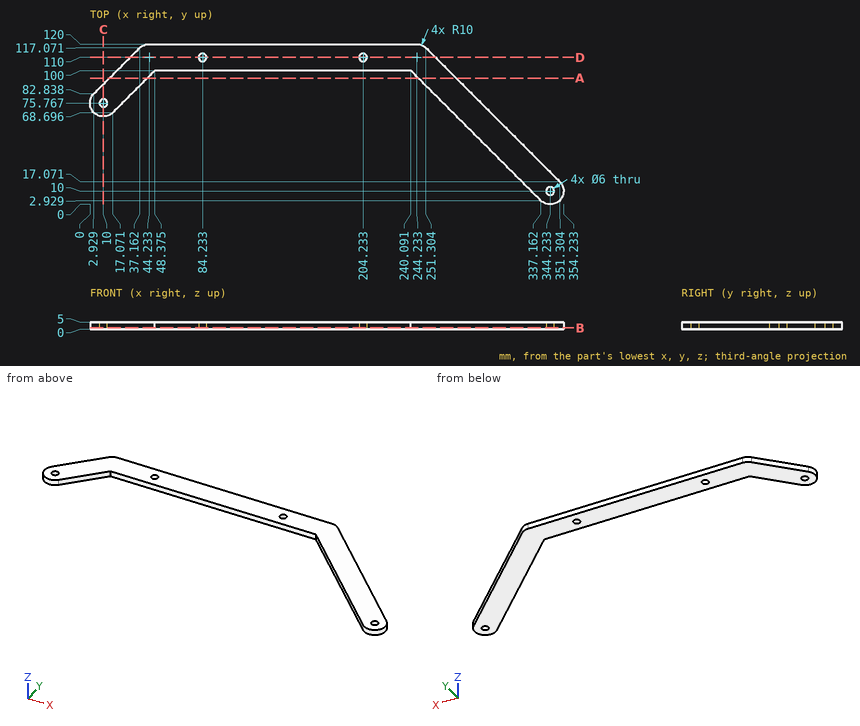
Geometry check sheet. Reference: drawing and pictorial views, mm from the part's lowest x, y, z. Round coordinates to 2 decimals unless told otherwise and drop trailing zeros. Loops run counter-clockwise (first coordinate to the right, second up) from the corner with the lowest first, then second, coordinate; pieces in that order, holes last.
1. Sectioned sample at B-B on z = 0.95. Record the boundary of the cut face in (x, y) (1 decimal), and give its area (3 significant figures).
2. Sectioned sample at D-D on y = 110. Record the boundary of the cut face in (x, z) (1 decimal).
3. Sectioned sample at A-A on y = 94.5. Record the boundary of the cut face in (x, z) (1 decimal), and give its area (3 significant figures).
4. Scan lines: probe 1 along Y at (x, z) = (53, 3.65); probe 2 along X at (y, z) = (87.5, 4.5) (1 decimal); probe 3 along Y at (x, z) = (10, 3.4). Record each from-to range of solid material in increasing order.
5. Sectioned sample at C-C on x = 10. Record the boundary of the cut face in (y, z), and give its area (3 significant figures).
6. Gauge pin test, flat ends, axial feed: pin 1 Ø3 at (x, z) = (152.5, 1) entering from -Y; pin 2 Ø3 at (y, z) = (71, 3.5) entering from -X; pin 3 Ø2 at (y, z) = (54, 3.5) entering from -X. Record the tip position at first contact, or that the pin passes through.
Recorded:
1. outline: (2.9, 82.8) arc R10 ccw to (17.1, 68.7) - (48.4, 100) - (240.1, 100) - (337.2, 2.9) arc R10 ccw to (351.3, 17.1) - (251.3, 117.1) arc R10 ccw to (244.2, 120) - (44.2, 120) arc R10 ccw to (37.2, 117.1) - close; hole circle Ø6 at (10, 75.8); hole circle Ø6 at (84.2, 110); hole circle Ø6 at (204.2, 110); hole circle Ø6 at (344.2, 10)
1. area: 7,990 mm2
2. outline: (30.1, 0) - (81.2, 0) - (81.2, 5) - (30.1, 5) - close; (87.2, 0) - (201.2, 0) - (201.2, 5) - (87.2, 5) - close; (207.2, 0) - (258.4, 0) - (258.4, 5) - (207.2, 5) - close
3. outline: (14.6, 0) - (42.9, 0) - (42.9, 5) - (14.6, 5) - close; (245.6, 0) - (273.9, 0) - (273.9, 5) - (245.6, 5) - close
3. area: 283 mm2
4. probe 1: y = 100 to 120
4. probe 2: x = 7.6 to 35.9, 252.6 to 280.9
4. probe 3: y = 65.77 to 72.77, 78.77 to 89.91
5. outline: (65.77, 0) - (72.77, 0) - (72.77, 5) - (65.77, 5) - close; (78.77, 0) - (89.91, 0) - (89.91, 5) - (78.77, 5) - close
5. area: 90.7 mm2
6. pin 1: stops at y = 100
6. pin 2: stops at x = 0.55
6. pin 3: stops at x = 285.09
